For this review, use the dimensioned drawing (mm, ordinates from the lowest corner) and the shaded views. A direction names the side the tool comes from. Round coordinates to 2 decimals unless told otherwise and drop trailing zeros. Loops run counter-clockwise (first coordinate to the right, second up) from the corner with the lowest first, then second, coordinate; pieces in that order, holes last. Notation, with made-up numbers: (24, 35.25) - (72, 35.25) arc R23 ccw to (72, 61.25) - close; hole circle Ø7 at (-23.75, 46.5). An arc over 180 degrees is marked (long way). Return JSON: item names as keys, results as strings. Group by question number.
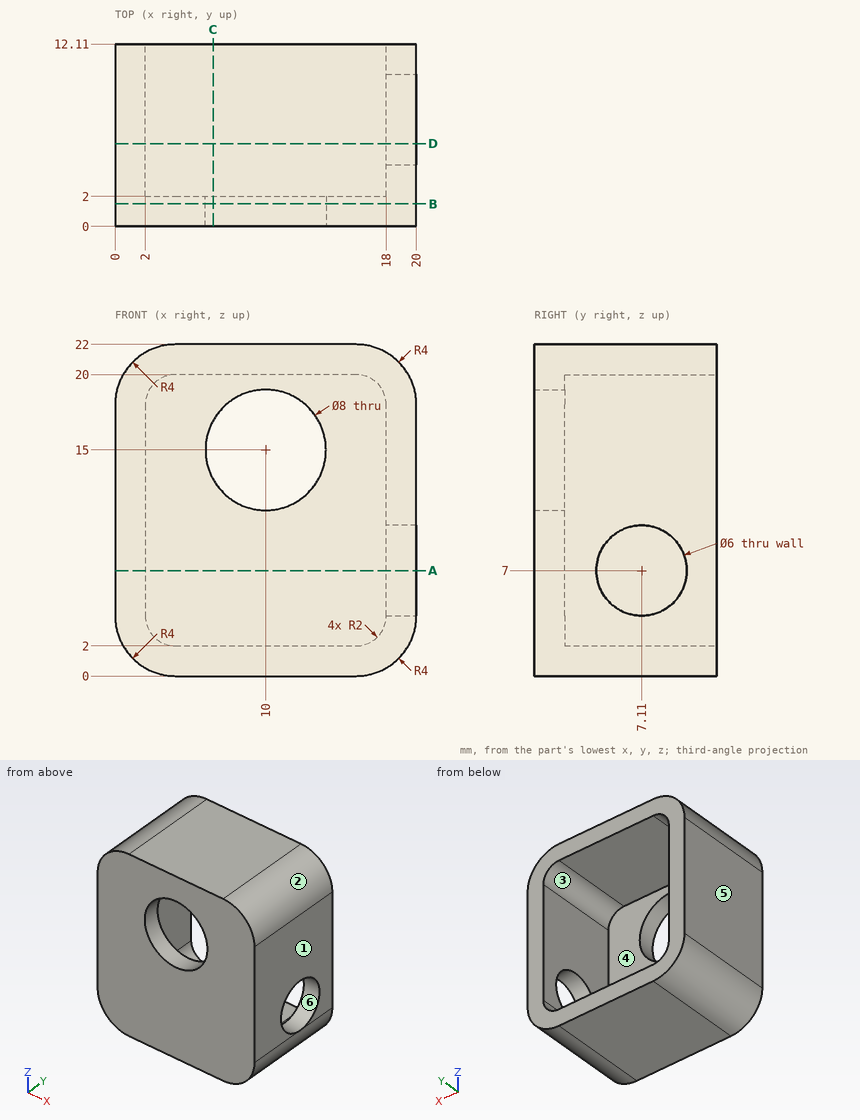
Q1. Add section D-D, the plane y = 5.5. State the section outline as (x, z) points.
Q2. Add section A-A, the plane z = 7. State the section outline as (x, y) points, plus the area to 3 significant figures.
Q3. Tool access review of the marked faces 4, 5 and 6: name each direction out of +Z, -Z, +X, -X, +Y, -Y from which nothing blocks a thin tool from reaching the whole face with its end or side.
Q4. Insertion check: pin 1 Ø5 at (x, z) = (12, 10.5) entering from +Y; pin 2 Ø6.5 at (x, z) = (10, 15) entering from +Y (3 decimals). Each pin has a flat end and moves straight along its axis. Give the tip position at first contact, or say it passes through.
Q5. Add section C-C, the plane x = 6.5. State the section outline as (y, z) points, plus the area to 3 significant figures.
Q6. Draft analysis for pull direction Z (two halves, no side actions). For the marked faces 1, 2 and 3, state which applies: pulls with the +Z half, pulls with the -Z half, needs draft (parallel to the pull), parting line crosses it, or undercut.
Q7. For line 1 (X direction, y = 2.75, z = 17.75); line 2 (Z direction, x = 13, y = 2.5); line 3 (Y direction, x = 19.3, z = 7), list the stretches that pass through material, from the lowest coordinate up.
Q8. Add section B-B, the plane y = 1.5. State the section outline as (x, z) points.
Evaluation:
{
 "1": {"outline": "(0, 4) arc R4 ccw to (4, 0) - (16, 0) arc R4 ccw to (20, 4) - (20, 4.47) - (18, 4.47) - (18, 4) arc R2 cw to (16, 2) - (4, 2) arc R2 cw to (2, 4) - (2, 18) arc R2 cw to (4, 20) - (16, 20) arc R2 cw to (18, 18) - (18, 9.53) - (20, 9.53) - (20, 18) arc R4 ccw to (16, 22) - (4, 22) arc R4 ccw to (0, 18) - close"},
 "2": {"outline": "(0, 0) - (20, 0) - (20, 4.11) - (18, 4.11) - (18, 2) - (2, 2) - (2, 12.11) - (0, 12.11) - close; (18, 10.11) - (20, 10.11) - (20, 12.11) - (18, 12.11) - close", "area": "68.4 mm²"},
 "3": {"face 4": "+Y", "face 5": "+Z, -Z, -X, +Y, -Y", "face 6": "+X"},
 "4": {"pin 1": "y = 2", "pin 2": "through"},
 "5": {"outline": "(0, 0) - (12.11, 0) - (12.11, 2) - (2, 2) - (2, 13.06) - (0, 13.06) - close; (0, 16.94) - (2, 16.94) - (2, 20) - (12.11, 20) - (12.11, 22) - (0, 22) - close", "area": "76.7 mm²"},
 "6": {"face 1": "needs draft", "face 2": "pulls with the +Z half", "face 3": "undercut"},
 "7": {"line 1": "0 to 2, 18 to 20", "line 2": "0 to 2, 20 to 22", "line 3": "0 to 4.11, 10.11 to 12.11"},
 "8": {"outline": "(0, 4) arc R4 ccw to (4, 0) - (16, 0) arc R4 ccw to (20, 4) - (20, 18) arc R4 ccw to (16, 22) - (4, 22) arc R4 ccw to (0, 18) - close; hole circle Ø8 at (10, 15)"}
}
